CAD build for the part. Positions are in the model's coordinates, mm. Give positions to 0.01 mm unless a question says otherwise; leave off trailing zeros. Loops run counter-clockwise (first coordinate to the right, second up) from the corner with the lowest first, then second, coordinate; pieces in that order, holes last. Notation, with made-up numbers: M 51.25,-5.5 L 96.25,-5.5 A14 cw 96.25,4.5 Z; hole C -39.75,-24 d3. An arc over 180 degrees is marked long. One line per question, with ' | ' between items.
```python
from build123d import *

# Parameters (mm, degrees)
F0_W     = 42
F0_H     = 62
F0_R     = 1.5
F0_R_2   = 11
F0_R_3   = 2.5
F1_DEPTH = 2
F2_SIZE  = 3
F3_R     = 2


with BuildPart() as f1:
    # F0 (on Top) → F1 (new body)
    with BuildSketch(Plane.XY):
        Rectangle(F0_W, F0_H)
        with Locations((-15.5, -25.5)):
            Circle(F0_R, mode=Mode.SUBTRACT)
        with Locations((15.5, -25.5)):
            Circle(F0_R, mode=Mode.SUBTRACT)
        with Locations((0, -10)):
            Circle(F0_R_2, mode=Mode.SUBTRACT)
        with Locations((-15.5, 5.5)):
            Circle(F0_R, mode=Mode.SUBTRACT)
        with Locations((-16, 21)):
            Circle(F0_R_3, mode=Mode.SUBTRACT)
        with Locations((15.5, 5.5)):
            Circle(F0_R, mode=Mode.SUBTRACT)
        with Locations((16, 21)):
            Circle(F0_R_3, mode=Mode.SUBTRACT)
    extrude(amount=F1_DEPTH)

    # F2
    f2_edges = [f1.edges().sort_by_distance(p)[0] for p in [
        (-21, -31, 1),
        (21, -31, 1),
    ]]
    chamfer(f2_edges, length=F2_SIZE)

    # F3
    f3_edges = [f1.edges().sort_by_distance(p)[0] for p in [
        (-18, -31, 1),
        (18, -31, 1),
        (21, -28, 1),
        (-21, -28, 1),
    ]]
    fillet(f3_edges, radius=F3_R)


solid = f1.part
```
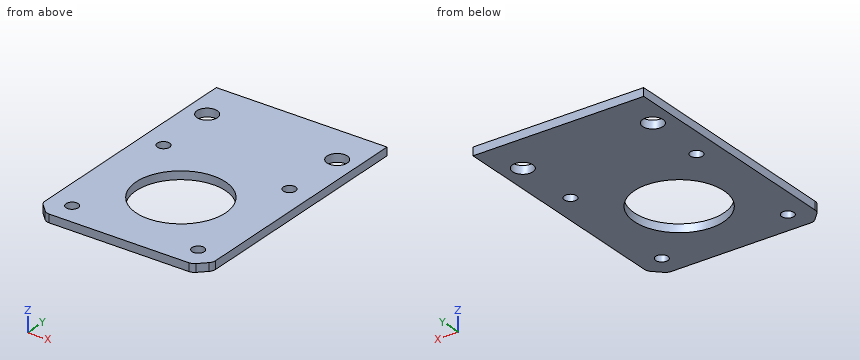
Item 1: Saw through at A-A on x = 0. Give the cut face in (y, z), and give its area (3 significant figures).
Conclusion:
outline: M -31,0 L -21,0 L -21,2 L -31,2 Z; M 1,0 L 31,0 L 31,2 L 1,2 Z | area: 80.0 mm²
Item 2: Drill centre lines: line 1 along Y through (x, z) = (-15.5, 1.65); line 2 along Y through (x, z) = (-15, 1.7); line 3 along Y through (x, z) = (-2.5, 0.55). Where is each one in solid material? Low to high. Write a range as [from, to].
Conclusion:
line 1: [-31, -27], [-24, 4], [7, 18.55], [23.45, 31] | line 2: [-31, -26.91], [-24.09, 4.09], [6.91, 18.71], [23.29, 31] | line 3: [-31, -20.71], [0.71, 31]
Item 3: Saw through at B-B on y = 21. Give the cut face in (x, z).
Conclusion:
outline: M -21,0 L -18.5,0 L -18.5,2 L -21,2 Z; M -13.5,0 L 13.5,0 L 13.5,2 L -13.5,2 Z; M 18.5,0 L 21,0 L 21,2 L 18.5,2 Z
Item 4: Saw through at D-D on x = 15.5. Give the cut face in (y, z).
Conclusion:
outline: M -31,0 L -27,0 L -27,2 L -31,2 Z; M -24,0 L 4,0 L 4,2 L -24,2 Z; M 7,0 L 18.55,0 L 18.55,2 L 7,2 Z; M 23.45,0 L 31,0 L 31,2 L 23.45,2 Z
Item 5: Saw through at C-C on z = 0.7. Give the cut face in (x, y), and give its area (3 significant figures).
Conclusion:
outline: M -21,-27.17 A2 ccw -20.41,-28.59 L -18.59,-30.41 A2 ccw -17.17,-31 L 17.17,-31 A2 ccw 18.59,-30.41 L 20.41,-28.59 A2 ccw 21,-27.17 L 21,31 L -21,31 Z; hole C -16,21 d5; hole C -15.5,-25.5 d3; hole C -15.5,5.5 d3; hole C 0,-10 d22; hole C 16,21 d5; hole C 15.5,-25.5 d3; hole C 15.5,5.5 d3 | area: 2,150 mm²
